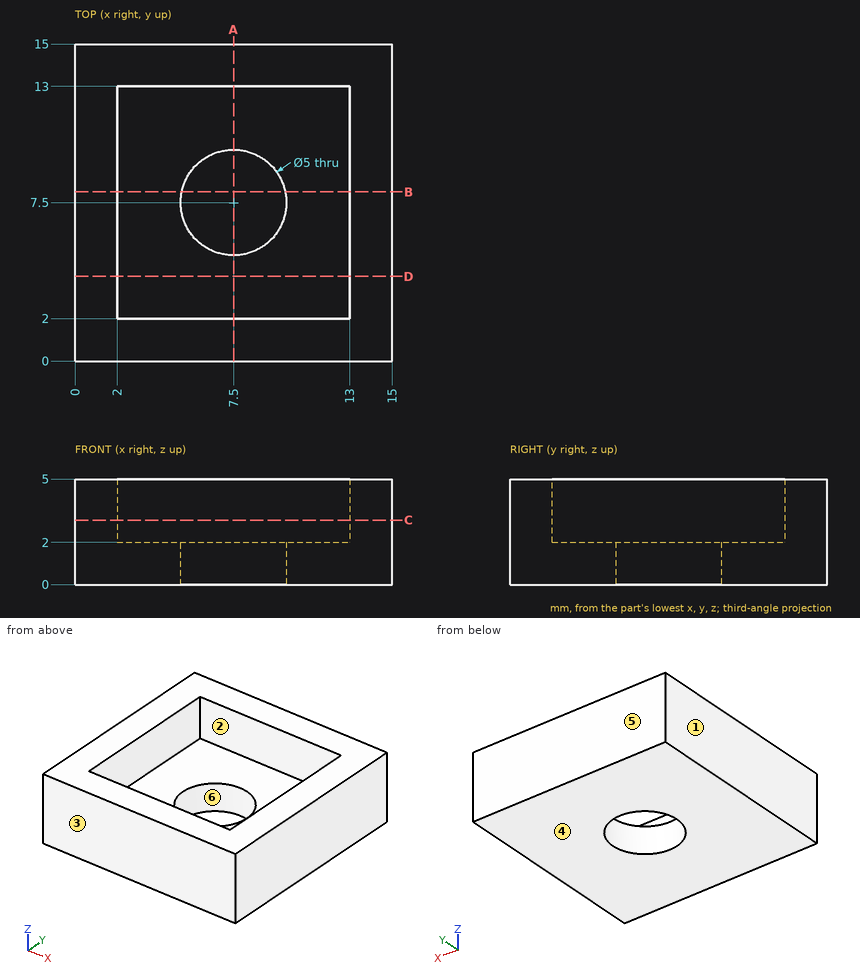
Could you check a few things on this drawing? It's one solid part, dimensions in mm from its lowest x, y, z. A direction names the side the tool comes from. Coordinates: 2 decimals unless noted, no trailing zeros. Order: outer loops, then holes, each group sorted by start corner. A loop starts at its lowest first (then second) coordinate and runs counter-clockwise, first axis right, second up.
1. Thinking about a two-plate mould opening in Y: for the marked faces 3, 4, 5 and 6, which applies, +Y half, -Y half, draft (parallel to the pull), parting line (faces both ways), or undercut?
2. If we section it at B-B (y = 8): Please give me the cut outline in (x, z).
3. If we section it at C-C (z = 3.05): Please give me the cut outline in (x, y).
4. For the marked faces 1 and 2, which set-ups out of +Z, -Z, +X, -X, +Y, -Y let a thin tool reach every point of the face, with its end or its side?
5. I need wall thicknesses on line 1 (Y direction, x = 11, z = 3.05); line 2 (Y direction, x = 7.5, z = 1). Which ranges of each line are inside material? Lowest first, please.
6. I'm going to push a flat-ended pin straight in: pin 1 (3.5 mm diameter, centred on x = 10, y = 7.5, fed in from +Z). Where does the tip first touch, or does it pass through?
7. If we section it at D-D (y = 4): Please give me the cut outline in (x, z).
8. If we section it at A-A (x = 7.5): Please give me the cut outline in (y, z), then the cut area to 3 significant figures.
Entries:
1. face 3: -Y half
1. face 4: draft
1. face 5: +Y half
1. face 6: undercut
2. outline: (0, 0) - (5.05, 0) - (5.05, 2) - (2, 2) - (2, 5) - (0, 5) - close; (9.95, 0) - (15, 0) - (15, 5) - (13, 5) - (13, 2) - (9.95, 2) - close
3. outline: (0, 0) - (15, 0) - (15, 15) - (0, 15) - close; hole (2, 2) - (13, 2) - (13, 13) - (2, 13) - close
4. face 1: +Z, -Z, -X, +Y, -Y
4. face 2: +Z
5. line 1: y = 0 to 2, 13 to 15
5. line 2: y = 0 to 5, 10 to 15
6. pin 1: stops at z = 2
7. outline: (0, 0) - (15, 0) - (15, 5) - (13, 5) - (13, 2) - (2, 2) - (2, 5) - (0, 5) - close
8. outline: (0, 0) - (5, 0) - (5, 2) - (2, 2) - (2, 5) - (0, 5) - close; (10, 0) - (15, 0) - (15, 5) - (13, 5) - (13, 2) - (10, 2) - close
8. area: 32.0 mm2
